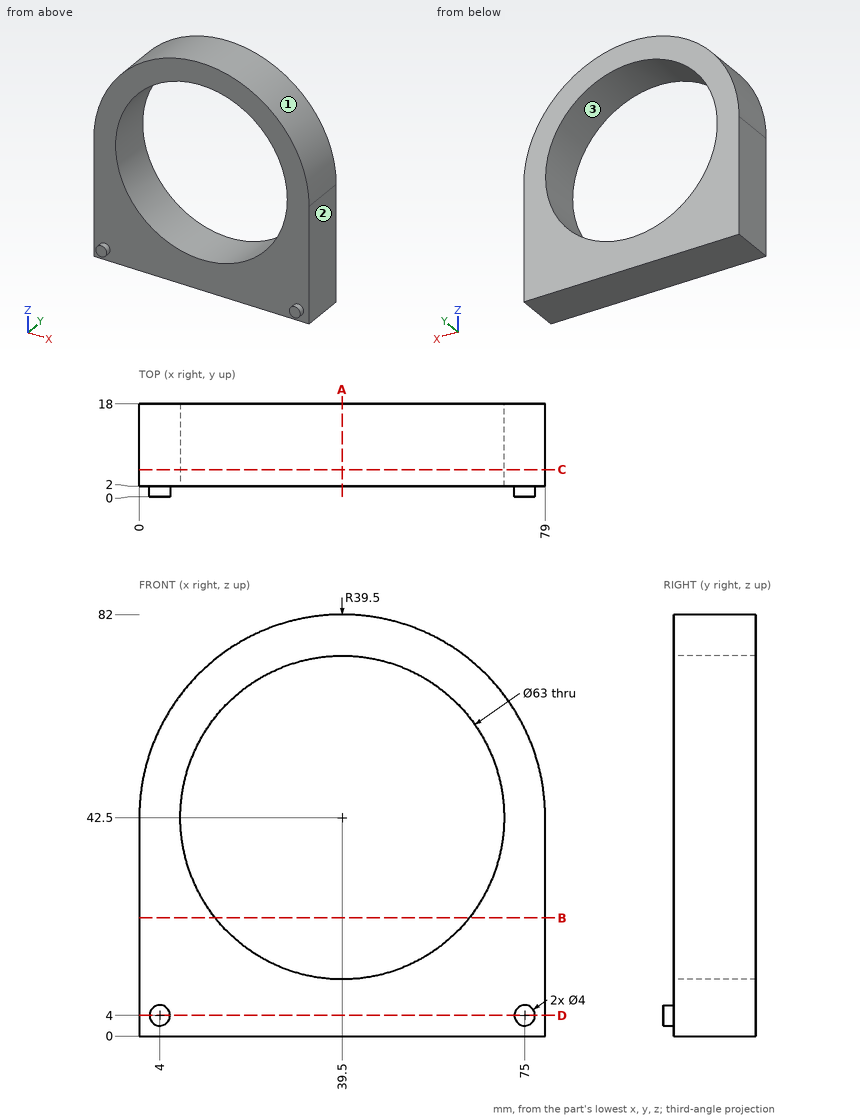
Study the drawing (mm; zero at the part's minimum x, y, z) and answer. Round coordinates to 2 decimals unless told otherwise and drop trailing zeros. Write each loop counter-clockwise with the first axis right and the second up, starting at its lowest first coordinate (ties: lowest second). Pieces come first, ordered by that corner, then holes.
Q1. Find section B-B on z = 23. Determine the outline of the cut face in (x, y).
Values:
outline: (0, 2) - (14.76, 2) - (14.76, 18) - (0, 18) - close; (64.24, 2) - (79, 2) - (79, 18) - (64.24, 18) - close
Q2. The mould has two halves that part along X. Classify the marked faces 1, 2 and 3: released by +X, released by -X, zero draft, split by the parting line, or undercut.
Values:
face 1: split by the parting line
face 2: released by +X
face 3: undercut
Q3. Find section C-C on y = 5.25. Determine the outline of the cut face in (x, z), and give its area (3 significant figures).
Values:
outline: (0, 0) - (79, 0) - (79, 42.5) arc R39.5 ccw to (0, 42.5) - close; hole circle Ø63 at (39.5, 42.5)
area: 2,690 mm2
Q4. Flat-ended cylindrical pins translate along their axes: P1, Ø8, axis at x = 33, y = 8.5, coming from the -Z side; P2, Ø3, axis at y = 5, z = 63, coming from the -X side; P3, Ø1, axis at y = 5.5, z = 50, coming from the -X side; P4, Ø4, axis at y = 11, z = 62.5, coming from the +X side. Find the tip coordinate at first contact, or state that the pin passes through.
Values:
P1: stops at z = 0
P2: stops at x = 4.87
P3: stops at x = 0.63
P4: stops at x = 74.66
Q5. Find section A-A on x = 39.5. Determine the outline of the cut face in (y, z), and give its area (3 significant figures).
Values:
outline: (2, 0) - (18, 0) - (18, 11) - (2, 11) - close; (2, 74) - (18, 74) - (18, 82) - (2, 82) - close
area: 304 mm2
Q6. Find section D-D on z = 4. Determine the outline of the cut face in (x, y).
Values:
outline: (0, 2) - (2, 2) - (2, 0) - (6, 0) - (6, 2) - (73, 2) - (73, 0) - (77, 0) - (77, 2) - (79, 2) - (79, 18) - (0, 18) - close
Q7. Straight lines are drawn through the part: line 1 (Z direction, x = 39.5, y = 10.25); line 2 (X direction, y = 8.5, z = 42.5); line 3 (X direction, y = 12.75, z = 71.5). For each, find the intervals that lie inside material, in ascending order.
Values:
line 1: z = 0 to 11, 74 to 82
line 2: x = 0 to 8, 71 to 79
line 3: x = 12.68 to 27.2, 51.8 to 66.32
